The listing builds one solid part. Answer for the finished solid, in the listing's coordinates (mm). Face numbers are marked on the shaded views. A direction names the side the tool comes from. Give positions to 0.01 mm unless a question says otherwise; leave off trailing zeros. Write each loop counter-clockwise with the first axis right and the second up, starting at its lowest first coordinate (ties: lowest second). Pieces come first, ordered by that corner, then holes. Notation, with made-up numbers: M -33,-1.5 L 21,-1.5 A9 cw 21,13.5 Z; hole C -19.5,-28 d1. An arc over 180 degrees is marked long. Return JSON: item names as keys, results as strings.
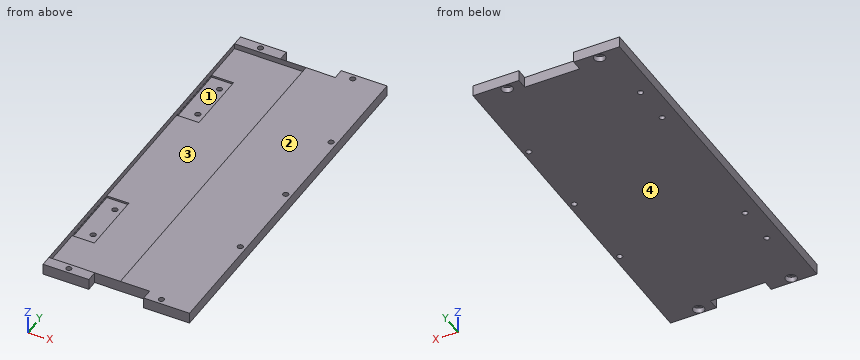
from build123d import *

# Parameters (mm, degrees)
ESQUISSE1_W             = 80
ESQUISSE1_H             = 200
BOSS_EXTRU_1_DEPTH      = 6
ESQUISSE4_W             = 39
ESQUISSE4_H             = 187.98
ENL_V_MAT_EXTRU_3_DEPTH = 3
ESQUISSE5_W             = 30
ESQUISSE5_H             = 6
ENL_V_MAT_EXTRU_4_DEPTH = 10
ESQUISSE6_R             = 2.995
ENL_V_MAT_EXTRU_5_DEPTH = 3
ESQUISSE7_R             = 1.5
ENL_V_MAT_EXTRU_6_DEPTH = 13
ESQUISSE8_R             = 1.5
ENL_V_MAT_EXTRU_7_DEPTH = 10
ESQUISSE9_R             = 1.5
ENL_V_MAT_EXTRU_8_DEPTH = 10
ESQUISSE10_W            = 12
ESQUISSE10_H            = 35
ENL_V_MAT_EXTRU_9_DEPTH = 1


with BuildPart() as part:
    # Esquisse1 → Boss.-Extru.1 (new body)
    with BuildSketch(Plane.XY):
        Rectangle(ESQUISSE1_W, ESQUISSE1_H)
    extrude(amount=BOSS_EXTRU_1_DEPTH)

    # Esquisse4 → Enlèv. mat.-Extru.3 (cut)
    with BuildSketch(Plane.XY.offset(6)):
        with Locations((-20.49, 0)):
            Rectangle(ESQUISSE4_W, ESQUISSE4_H)
    extrude(amount=-ENL_V_MAT_EXTRU_3_DEPTH, mode=Mode.SUBTRACT)

    # Esquisse5 → Enlèv. mat.-Extru.4 (cut)
    with BuildSketch(Plane.XY.offset(6)):
        with Locations((0, 97)):
            Rectangle(ESQUISSE5_W, ESQUISSE5_H)
        with Locations((0, -97)):
            Rectangle(ESQUISSE5_W, ESQUISSE5_H)
    extrude(amount=-ENL_V_MAT_EXTRU_4_DEPTH, mode=Mode.SUBTRACT)

    # Esquisse6 → Enlèv. mat.-Extru.5 (cut)
    with BuildSketch(Plane(origin=(0, 0, 0), x_dir=(-1, 0, 0), z_dir=(0, 0, -1))):
        with Locations((27.5, -97)):
            Circle(ESQUISSE6_R)
        with Locations((-23, -97)):
            Circle(ESQUISSE6_R)
        with Locations((27.5, 97)):
            Circle(ESQUISSE6_R)
        with Locations((-23, 97)):
            Circle(ESQUISSE6_R)
    extrude(amount=-ENL_V_MAT_EXTRU_5_DEPTH, mode=Mode.SUBTRACT)

    # Esquisse7 → Enlèv. mat.-Extru.6 (cut)
    with BuildSketch(Plane(origin=(0, 0, 0), x_dir=(-1, 0, 0), z_dir=(0, 0, -1))):
        with Locations((27.5, 97)):
            Circle(ESQUISSE7_R)
        with Locations((-22.909579605, 97)):
            Circle(ESQUISSE7_R)
        with Locations((27.5, -97)):
            Circle(ESQUISSE7_R)
        with Locations((-23, -97)):
            Circle(ESQUISSE7_R)
    extrude(amount=-ENL_V_MAT_EXTRU_6_DEPTH, mode=Mode.SUBTRACT)

    # Esquisse8 → Enlèv. mat.-Extru.7 (cut)
    with BuildSketch(Plane.XY.offset(3)):
        with Locations((-32.01, 64)):
            Circle(ESQUISSE8_R)
        with Locations((-32.01, 42)):
            Circle(ESQUISSE8_R)
        with Locations((-32.01, -42)):
            Circle(ESQUISSE8_R)
        with Locations((-32.01, -64)):
            Circle(ESQUISSE8_R)
    extrude(amount=-ENL_V_MAT_EXTRU_7_DEPTH, mode=Mode.SUBTRACT)

    # Esquisse9 → Enlèv. mat.-Extru.8 (cut)
    with BuildSketch(Plane(origin=(0, 0, 0), x_dir=(-1, 0, 0), z_dir=(0, 0, -1))):
        with Locations((-37, -43)):
            Circle(ESQUISSE9_R)
        with Locations((-37, 3)):
            Circle(ESQUISSE9_R)
        with Locations((-37, 49)):
            Circle(ESQUISSE9_R)
    extrude(amount=-ENL_V_MAT_EXTRU_8_DEPTH, mode=Mode.SUBTRACT)

    # Esquisse10 → Enlèv. mat.-Extru.9 (cut)
    with BuildSketch(Plane.XY.offset(3)):
        with Locations((-33.9, 53)):
            Rectangle(ESQUISSE10_W, ESQUISSE10_H)
        with Locations((-33.9, -53)):
            Rectangle(ESQUISSE10_W, ESQUISSE10_H)
    extrude(amount=-ENL_V_MAT_EXTRU_9_DEPTH, mode=Mode.SUBTRACT)


solid = part.part
Item 1: Determine the mould class of the marked faces 3 and 4 for opening direction X: +X half, -X half, draft (parallel to the pull), parting line (faces both ways), or undercut.
Geometry results:
{"face 3": "undercut", "face 4": "draft"}
Item 2: Find the intervals of material crossed by line 1 (Y direction, x = -27.5, z = 4.7); line 2 (Y direction, x = -32.01, z = 1.15); line 3 (Y direction, x = -31, z = 2.95), in increasing order.
Geometry results:
{"line 1": "y = -100 to -98.5, -95.5 to -93.99, 93.99 to 95.5, 98.5 to 100", "line 2": "y = -100 to -65.5, -62.5 to -43.5, -40.5 to 40.5, 43.5 to 62.5, 65.5 to 100", "line 3": "y = -100 to -70.5, -35.5 to 35.5, 70.5 to 100"}
Item 3: Given pin 1 Ø3.5 at (x, y) = (22.91, 97) entering from -Z, flat-ended and moving along its own axis, determine where the tip first touches the part or whether it passes through.
Geometry results:
{"pin 1": "stops at z = 3"}
Item 4: A cutting plane is placed at D-D, the plane x = 1.5. Write down the section's boundary in (y, z), plus the area to 3 significant figures.
Geometry results:
{"outline": "M -94,0 L 94,0 L 94,6 L -94,6 Z", "area": "1,130 mm2"}
Item 5: A cutting plane is placed at A-A, the plane z = 4.95. Count the separate pieces of the cut face and the enclosed holes in it, plus the area to 3 significant figures.
Geometry results:
{"separate pieces": "1", "enclosed holes": "8", "area": "8,260 mm2"}
Item 6: Which of the six approach directions +Z, -Z, +X, -X, +Y, -Y give full straight-line access (tool end or side, diameter ignored) to the marked faces 1 and 2?
Geometry results:
{"face 1": "+Z", "face 2": "+Z, +X, -X, +Y, -Y"}
